from build123d import *

# Parameters (mm, degrees)
CROQUIS1_W                = 112
CROQUIS1_H                = 112
SALIENTE_EXTRUIR1_DEPTH   = 10
CROQUIS2_R                = 4
CORTAR_EXTRUIR1_DEPTH     = 6
CROQUIS3_R                = 4
CORTAR_EXTRUIR2_DEPTH     = 6
SIMETR_A2_COPY_1_SKETCH_R = 4
SIMETR_A2_COPY_1_DEPTH    = 6
SIMETR_A2_COPY_2_SKETCH_R = 4
SIMETR_A2_COPY_2_DEPTH    = 6


with BuildPart() as part:
    # Croquis1 → Saliente-Extruir1 (new body)
    with BuildSketch(Plane.XY):
        with Locations((56, 56)):
            Rectangle(CROQUIS1_W, CROQUIS1_H)
        Polygon((20, 10), (92, 10), (92, 20), (102, 20), (102, 92), (92, 92), (92, 102), (20, 102), (20, 92), (10, 92), (10, 20), (20, 20), align=None, mode=Mode.SUBTRACT)
    extrude(amount=SALIENTE_EXTRUIR1_DEPTH)

    # Croquis2 → Cortar-Extruir1 (cut)
    with BuildSketch(Plane.XZ.offset(-92)):
        with Locations((97, 5)):
            Circle(CROQUIS2_R)
    cortar_extruir1 = extrude(amount=-CORTAR_EXTRUIR1_DEPTH, mode=Mode.SUBTRACT)

    # Croquis3 → Cortar-Extruir2 (cut)
    with BuildSketch(Plane.ZY.offset(-92)):
        with Locations((5, 97)):
            Circle(CROQUIS3_R)
    cortar_extruir2 = extrude(amount=-CORTAR_EXTRUIR2_DEPTH, mode=Mode.SUBTRACT)

    # Simetría1: Cortar-Extruir1, Cortar-Extruir2 across plane
    add(cortar_extruir1.mirror(Plane.ZY.offset(-56)), mode=Mode.SUBTRACT)
    add(cortar_extruir2.mirror(Plane.ZY.offset(-56)), mode=Mode.SUBTRACT)

    # Simetría2: Cortar-Extruir1, Cortar-Extruir2 across plane
    add(cortar_extruir1.mirror(Plane.ZX.offset(56)), mode=Mode.SUBTRACT)
    add(cortar_extruir2.mirror(Plane.ZX.offset(56)), mode=Mode.SUBTRACT)

    # Simetría2 copy 1 sketch → Simetría2 copy 1 (cut)
    with BuildSketch(Plane(origin=(112, 20, 0), x_dir=(-1, 0, 0), z_dir=(0, 1, 0))):
        with Locations((97, 5)):
            Circle(SIMETR_A2_COPY_1_SKETCH_R)
    extrude(amount=-SIMETR_A2_COPY_1_DEPTH, mode=Mode.SUBTRACT)

    # Simetría2 copy 2 sketch → Simetría2 copy 2 (cut)
    with BuildSketch(Plane(origin=(20, 112, 0), x_dir=(0, 0, 1), z_dir=(1, 0, 0))):
        with Locations((5, 97)):
            Circle(SIMETR_A2_COPY_2_SKETCH_R)
    extrude(amount=-SIMETR_A2_COPY_2_DEPTH, mode=Mode.SUBTRACT)


solid = part.part
Source: CAD feature listing. Evaluate the final solid. Frame: model axes, mm. A direction names the side the tool comes from. Round coordinates to 2 decimals unless told otherwise and drop trailing zeros. Write each loop counter-clockwise with the first axis right and the second up, starting at its lowest first coordinate (ties: lowest second). Pieces come first, ordered by that corner, then holes. Notation, with made-up numbers: (77, 9.25) - (91, 9.25) arc R20 cw to (91, 18.25) - close; hole circle Ø5 at (-32.5, 31). An arc over 180 degrees is marked (long way). Use CSV: the item, a comma, the result in double quotes. Start each with the question number.
(1) Material intervals for probe 1 along X at (y, z) = (63, 1.5); probe 2 along Y at (x, z) = (93.5, 5); probe 3 along Y at (x, z) = (100.5, 6), sorted ascending. Write a range as [from, to].
(2) Cut plane C-C, the plane z = 5. Give the number of separate pieces and of enclosed holes in the cut face, and give its area (3 significant figures).
(3) Cut plane A-A, the plane x = 33. Return loops of the section in (y, z), and give its area (3 significant figures).
(4) Mould query, pull axis Y, two halves, no side actions, for faces 1 (the face through (5, 57, 10)), 2 (the face through (102, 55, 5)). Classes: pulls with the +Y half, pulls with the -Y half, needs draft (parallel to the pull), parting line crosses it, or undercut.
(5) Set-up query: faces 3 (the face through (112, 55, 5)), 4 (the face through (20, 19.5, 4.9)), 5 (the face through (14, 13, 5)). Return all of +Z, -Z, +X, -X, +Y, -Y with unobstructed straight access to the full face (end or side cutting, diameter ignored); none if empty.
Geometry says:
1,probe 1,"[0, 10], [102, 112]"
1,probe 2,"[0, 11], [101, 112]"
1,probe 3,"[0, 14], [98, 112]"
2,separate pieces,"5"
2,enclosed holes,"1"
2,area,"4,200 mm²"
3,outline,"(0, 0) - (10, 0) - (10, 10) - (0, 10) - close; (102, 0) - (112, 0) - (112, 10) - (102, 10) - close"
3,area,"200 mm²"
4,face 1,"needs draft"
4,face 2,"undercut"
5,face 3,"+Z, -Z, +X, +Y, -Y"
5,face 4,"+Z, -Z"
5,face 5,"none"
